```python
from build123d import *

# Parameters (mm, degrees)
SKETCH1_R                = 8
SKETCH1_R_2              = 2.5
BOSS_EXTRUDE1_DEPTH      = 11.25
SKETCH2_R                = 3.175
CUT_EXTRUDE1_DEPTH       = 11.25
SKETCH3_R                = 8
BOSS_EXTRUDE2_DEPTH      = 4.9
BOSS_EXTRUDE2_DEPTH_BACK = 4.9


with BuildPart() as part:
    # Sketch1 → Boss-Extrude1 (new body, symmetric)
    with BuildSketch(Plane(origin=(0, 0, 0), x_dir=(0, 0, -1), z_dir=(1, 0, 0))):
        Circle(SKETCH1_R)
        Circle(SKETCH1_R_2, mode=Mode.SUBTRACT)
    extrude(amount=BOSS_EXTRUDE1_DEPTH, both=True)

    # Sketch2 → Cut-Extrude1 (cut)
    with BuildSketch(Plane(origin=(11.25, 0, 0), x_dir=(0, 0, -1), z_dir=(1, 0, 0))):
        Circle(SKETCH2_R)
    extrude(amount=-CUT_EXTRUDE1_DEPTH, mode=Mode.SUBTRACT)

    # Sketch3 → Boss-Extrude2 (add, two sides)
    with BuildSketch(Plane(origin=(0, 0, 0), x_dir=(0, 0, -1), z_dir=(1, 0, 0))) as boss_extrude2_sk:
        Circle(SKETCH3_R)
    extrude(amount=BOSS_EXTRUDE2_DEPTH)
    extrude(boss_extrude2_sk.sketch, amount=-BOSS_EXTRUDE2_DEPTH_BACK)


solid = part.part
```
Build history of the part. All positions in model axes, mm. A direction names the side the tool comes from. Round coordinates to 2 decimals unless told otherwise and drop trailing zeros. Write each loop counter-clockwise with the first axis right and the second up, starting at its lowest first coordinate (ties: lowest second). Pieces come first, ordered by that corner, then holes. Notation, with made-up numbers: (47.25, 7.5) - (106.25, 7.5) arc R14 ccw to (106.25, 14.5) - close; hole circle Ø1 at (73, 8.25). An arc over 180 degrees is marked (long way). Answer as CSV lines item,"result".
Q1. Cut at A-A (y = 0). Write the cut outline in (x, z) (3 decimals).
Report:
outline,"(-11.25, -8) - (11.25, -8) - (11.25, -3.175) - (4.9, -3.175) - (4.9, 3.175) - (11.25, 3.175) - (11.25, 8) - (-11.25, 8) - (-11.25, 2.5) - (-4.9, 2.5) - (-4.9, -2.5) - (-11.25, -2.5) - close"
Q2. Cut at C-C (x = -8.75). Write the cut outline in (y, z).
Report:
outline,"circle Ø16 at (0, 0); hole circle Ø5 at (0, 0)"
Q3. Drop flat-ended pins along their axis: pin 1 (4 mm diameter, centred on x = 5.5, y = -0.5, fed in from -Z); pin 2 (5 mm diameter, centred on x = 9, y = -5.5, fed in from +Z); pin 3 (3 mm diameter, centred on y = 0, z = 0, fed in from +X); pin 4 (8 mm diameter, centred on x = 7.5, z = -5.5, fed in from -Y). Give the stop position or say it passes through.
Report:
pin 1,"stops at z = -8"
pin 2,"stops at z = 7.42"
pin 3,"stops at x = 4.9"
pin 4,"stops at y = -7.86"
Q4. Pull direction Y, two halves, no side cores. Call faces 4 (the cylindrical face through (0.16, -7.81, 1.73)), 5 (the cylindrical face through (8.12, -3.1, 0.69)), 6 (the flat face through (11.25, 0.1, -3.4)): +Y half, -Y half, draft (parallel to the pull), parting line (faces both ways), or undercut.
Report:
face 4,"parting line"
face 5,"undercut"
face 6,"draft"
Q5. Tool access for faces 1 (the flat face through (4.9, 0, 0)), 2 (the cylindrical face through (-8.12, -2.44, 0.54)), 3 (the flat face through (-11.25, 2, -2)): list every direction of +Z, -Z, +X, -X, +Y, -Y with a clear straight run to the whole face (end or side of a thin tool).
Report:
face 1,"+X"
face 2,"-X"
face 3,"+Z, -Z, -X, +Y, -Y"
Q6. Drill centre lines: probe 1 along Y at (x, z) = (-9, 0); probe 2 along X at (y, z) = (-0.75, 2.25); probe 3 along Z at (x, y) = (6.25, 7.25). Where is each one in solid material? Low to high. Write a range as [from, to].
Report:
probe 1,"y = [-8, -2.5], [2.5, 8]"
probe 2,"x = [-4.9, 4.9]"
probe 3,"z = [-3.38, 3.38]"
Q7. Cut at D-D (z = 7.25). Write the cut outline in (x, y), and give its area (3 significant figures).
Report:
outline,"(-11.25, -3.38) - (11.25, -3.38) - (11.25, 3.38) - (-11.25, 3.38) - close"
area,"152 mm^2"
